Can you work these out from the model? Positions are in its coordinate system, mm. Face numbers are marked on the shaded views. A direction names the side the tool comes from. Coordinates: 2 decimals unless noted, no trailing zeros. Loops run counter-clockwise (first coordinate to the right, second up) from the corner with the lowest first, then second, coordinate; pieces in that order, holes last. Notation, with made-up numbers: (4.5, -39.75) -> (35.5, -39.75) arc R11 ccw to (35.5, -23.75) -> close; hole circle Ø11 at (18, -19). An arc over 180 degrees is marked (long way). Use one line per item in the form item = value. Start each with the question number.
(1) I need wall thicknesses on line 1 (Y direction, x = 7.5, z = 7.5); line 2 (X direction, y = -8, z = 4.5); line 3 (X direction, y = -23.5, z = 2). Which ranges of each line are inside material? Lowest first, please. Write a range as [from, to].
(2) Thinking about a two-plate mould opening in Y: for the marked faces 1, 2, 3 and 4, which applies, released by +Y, released by -Y, zero draft, split by the parting line, or undercut?
(3) Imagine slicing it at C-C (x = -7). List the corners of the cut face in (y, z) for me (3 decimals).
(4) On a 3-axis mill with a long thin cutter (end or side, diameter ignored), from which of +Z, -Z, +X, -X, +Y, -Y can I reach the whole of each face in a straight line? I mean the marked faces 5, 6 and 7. Say none if no direction works.
(5) Imagine slicing it at D-D (y = -34.5). List the corners of the cut face in (x, z) for me, plus the area to 3 significant figures.
(6) I'm going to push flat-ended pins straight in: pin 1 (3 mm diameter, centred on y = -35.5, z = 6, fed in from -X); pin 2 (5 mm diameter, centred on x = 9, z = 7.5, fed in from -Y); pin 3 (3 mm diameter, centred on x = -10.5, z = 8.5, fed in from +Y); pin 4 (4 mm diameter, centred on x = -37, z = 10, fed in from -Y) (3 decimals). Where does each tip first touch, or does it pass through?
(7) Imagine slicing it at B-B (y = -1). List the corners of the cut face in (x, z) for me, plus the area to 3 significant figures.
(8) Imagine slicing it at A-A (x = 4.5). List the corners of the cut face in (y, z) for me.
```python
from build123d import *

# Parameters (mm, degrees)
BOSS_EXTRUDE2_DEPTH = 11.43
SKETCH4_W           = 20.955
SKETCH4_H           = 12.7
CUT_EXTRUDE2_DEPTH  = 1.016
SKETCH5_R           = 2.25
CUT_EXTRUDE3_DEPTH  = 66.915251214
SKETCH6_R           = 1.524
CUT_EXTRUDE4_DEPTH  = 76.777894678
SKETCH7_W           = 11.43
SKETCH7_H           = 11.049
CUT_EXTRUDE5_DEPTH  = 4.826
SKETCH8_W           = 6.35
SKETCH8_H           = 6.35
CUT_EXTRUDE6_DEPTH  = 12.914
SKETCH9_R           = 5.715
CUT_EXTRUDE7_DEPTH  = 5.548
CUT_EXTRUDE8_DEPTH  = 66.915251214
FILLET1_R           = 1.27
FILLET2_R           = 2.54
FILLET3_R           = 5.715


with BuildPart() as part:
    # Sketch1 → Boss-Extrude2 (new body)
    with BuildSketch(Plane.XY):
        Polygon((13.0175, 0), (13.0175, 44.6024), (-13.6525, 44.6024), (-13.6525, 15.875), (-47.1678, 15.875), (-47.1678, 0), (-47.1678, -15.875), (-13.6525, -15.875), (-13.6525, -44.6024), (13.0175, -44.6024), align=None)
        Polygon((-5.7658, 27.4574), (-5.7658, -27.4574), (-2.997199182, -27.4574), (-2.997199182, -18.0721), (5.7658, -18.0721), (5.7658, 18.0721), (-2.997199182, 18.0721), (-2.997199182, 27.4574), align=None, mode=Mode.SUBTRACT)
    extrude(amount=BOSS_EXTRUDE2_DEPTH)

    # Sketch4 → Cut-Extrude2 (cut)
    with BuildSketch(Plane.XY.offset(11.43)):
        with Locations((0, 35.7124)):
            Rectangle(SKETCH4_W, SKETCH4_H)
        with Locations((0, -35.7124)):
            Rectangle(SKETCH4_W, SKETCH4_H)
    extrude(amount=-CUT_EXTRUDE2_DEPTH, mode=Mode.SUBTRACT)

    # Sketch5 → Cut-Extrude3 (cut, through all)
    with BuildSketch(Plane.XY.offset(11.43)):
        with Locations((-40.1828, 8.255)):
            Circle(SKETCH5_R)
        with Locations((-23.6728, -8.255)):
            Circle(SKETCH5_R)
    extrude(amount=-CUT_EXTRUDE3_DEPTH, mode=Mode.SUBTRACT)

    # Sketch6 → Cut-Extrude4 (cut, through all)
    with BuildSketch(Plane(origin=(13.0175, 0, 0), x_dir=(0, 0, -1), z_dir=(1, 0, 0))):
        with Locations((-5.715, 22.767528581)):
            Circle(SKETCH6_R)
        with Locations((-5.715, -22.767528581)):
            Circle(SKETCH6_R)
    extrude(amount=-CUT_EXTRUDE4_DEPTH, mode=Mode.SUBTRACT)

    # Sketch7 → Cut-Extrude5 (cut)
    with BuildSketch(Plane.ZY.offset(13.6525)):
        with Locations((5.715, 21.3995)):
            Rectangle(SKETCH7_W, SKETCH7_H)
        with Locations((5.715, -21.3995)):
            Rectangle(SKETCH7_W, SKETCH7_H)
    extrude(amount=-CUT_EXTRUDE5_DEPTH, mode=Mode.SUBTRACT)

    # Sketch8 → Cut-Extrude6 (cut)
    with BuildSketch(Plane(origin=(13.0175, 0, 0), x_dir=(0, 0, -1), z_dir=(1, 0, 0))):
        with Locations((-5.715, -22.767528581)):
            Rectangle(SKETCH8_W, SKETCH8_H)
        with Locations((-5.715, 22.767528581)):
            Rectangle(SKETCH8_W, SKETCH8_H)
    extrude(amount=-CUT_EXTRUDE6_DEPTH, mode=Mode.SUBTRACT)

    # Sketch9 → Cut-Extrude7 (cut)
    with BuildSketch(Plane.XY):
        with Locations((-40.1828, 8.255)):
            Circle(SKETCH9_R)
        with Locations((-23.6728, -8.255)):
            Circle(SKETCH9_R)
    extrude(amount=CUT_EXTRUDE7_DEPTH, mode=Mode.SUBTRACT)

    # Sketch10 → Cut-Extrude8 (cut, through all)
    with BuildSketch(Plane.XY.offset(11.43)):
        Polygon((-2.747199182, 27.7074), (-6.015799182, 27.7074), (-6.015799182, -27.7074), (-2.747199182, -27.7074), (-2.747199182, -18.3221), (6.015800818, -18.3221), (6.015800818, 18.3221), (-2.747199182, 18.3221), align=None)
        Polygon((-2.997199182, 27.4574), (-5.765799182, 27.4574), (-5.765799182, -27.4574), (-2.997199182, -27.4574), (-2.997199182, -18.0721), (5.7658, -18.0721), (5.765800818, 18.0721), (-2.997199182, 18.0721), align=None, mode=Mode.SUBTRACT)
    extrude(amount=-CUT_EXTRUDE8_DEPTH, mode=Mode.SUBTRACT)


with BuildPart() as cut_extrude8_kept_piece:
    # of the separate pieces the step leaves, the one the design keeps (cut_extrude8_pieces_kept)
    add(part.part.solids().sort_by_distance((13.0175, 44.6024, 0))[0])

    # Fillet1
    fillet1_edges = [cut_extrude8_kept_piece.edges().sort_by_distance(p)[0] for p in [
        (-13.6525, 26.924, 5.715),
        (-8.8265, 26.924, 5.715),
        (-8.8265, 15.875, 5.715),
        (-13.6525, -26.924, 5.715),
        (-8.8265, -26.924, 5.715),
        (-8.8265, -15.875, 5.715),
    ]]
    fillet(fillet1_edges, radius=FILLET1_R)

    # Fillet2
    fillet2_edges = [cut_extrude8_kept_piece.edges().sort_by_distance(p)[0] for p in [
        (-47.1678, -15.875, 5.715),
        (-47.1678, 15.875, 5.715),
    ]]
    fillet(fillet2_edges, radius=FILLET2_R)

    # Fillet3
    fillet3_edges = [cut_extrude8_kept_piece.edges().sort_by_distance(p)[0] for p in [
        (13.0175, -44.6024, 5.715),
        (-13.6525, -44.6024, 5.715),
        (-13.6525, 44.6024, 5.715),
        (13.0175, 44.6024, 5.715),
    ]]
    fillet(fillet3_edges, radius=FILLET3_R)


solid = cut_extrude8_kept_piece.part
```
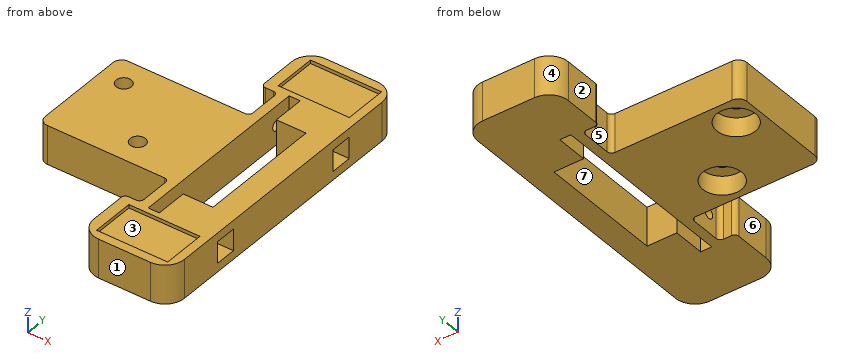
Worked out:
q1.line_1 = [-44.6, -25.94], [-19.59, 19.59], [25.94, 44.6]
q1.line_2 = [-47.17, -29.38], [-17.96, -6.02], [6.02, 13.02]
q1.line_3 = [-8.83, -6.02], [-2.75, 13.02]
q2.face_1 = released by -Y
q2.face_2 = zero draft
q2.face_3 = undercut
q2.face_4 = released by +Y
q3.outline = (-44.602, 0) -> (44.602, 0) -> (44.602, 11.43) -> (42.062, 11.43) -> (42.062, 10.414) -> (29.362, 10.414) -> (29.362, 11.43) -> (-29.362, 11.43) -> (-29.362, 10.414) -> (-42.062, 10.414) -> (-42.062, 11.43) -> (-44.602, 11.43) -> close; hole circle Ø3.048 at (-22.768, 5.715); hole circle Ø3.048 at (22.768, 5.715)
q4.face_5 = +Z, -Z, -X
q4.face_6 = +Z, -Z, -X, -Y
q4.face_7 = +Z, -Z
q5.outline = (-13.65, 0) -> (13.02, 0) -> (13.02, 11.43) -> (10.48, 11.43) -> (10.48, 10.41) -> (-10.48, 10.41) -> (-10.48, 11.43) -> (-13.65, 11.43) -> close
q5.area = 284 mm2
q6.pin_1 = -13.65
q6.pin_2 = -44.6
q6.pin_3 = 44.5
q6.pin_4 = -15.875
q7.outline = (-47.17, 0) -> (-6.02, 0) -> (-6.02, 11.43) -> (-47.17, 11.43) -> close; (6.02, 0) -> (13.02, 0) -> (13.02, 11.43) -> (6.02, 11.43) -> close
q7.area = 550 mm2
q8.outline = (-44.6, 0) -> (-18.32, 0) -> (-18.32, 11.43) -> (-29.36, 11.43) -> (-29.36, 10.41) -> (-42.06, 10.41) -> (-42.06, 11.43) -> (-44.6, 11.43) -> close; (18.32, 0) -> (44.6, 0) -> (44.6, 11.43) -> (42.06, 11.43) -> (42.06, 10.41) -> (29.36, 10.41) -> (29.36, 11.43) -> (18.32, 11.43) -> close; hole (-25.94, 2.54) -> (-19.59, 2.54) -> (-19.59, 8.89) -> (-25.94, 8.89) -> close; hole (19.59, 2.54) -> (25.94, 2.54) -> (25.94, 8.89) -> (19.59, 8.89) -> close
